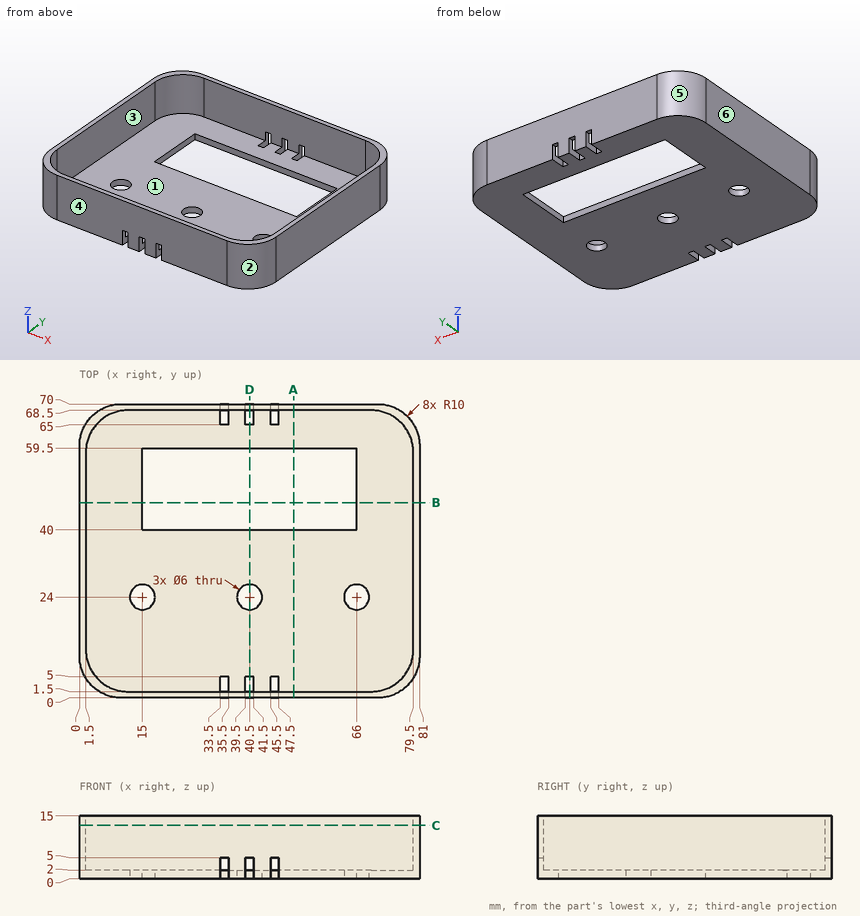
Job drawing, mm, ordinate dimensions from the low corner. One solid piece. A direction names the side the tool comes from. Coordinates: 2 decimals unless noted, no trailing zeros. Order: outer loops, then holes, each group sorted by start corner. A loop starts at its lowest first (then second) coordinate and runs counter-clockwise, first axis right, second up. Notation, with made-up numbers: (39.25, -30) -> (71.25, -30) arc R25 cw to (71.25, -9) -> close; hole circle Ø6 at (13.25, 66.5). An arc over 180 degrees is marked (long way). Return JSON: item names as keys, results as strings. Group by question number.
Item 1: Pull direction Y, two halves, no side cores. Call the marked faces 3, 4, 5 and 6: pulls with the +Y half, pulls with the -Y half, needs draft (parallel to the pull), parting line crosses it, or undercut.
Item 2: Saw through at C-C on z = 12.75. Write the cut outline in (x, y).
Item 3: Saw through at B-B on y = 46.5. Write the cut outline in (x, z).
Item 4: Wall check: line 1 along Y through (x, z) = (40.5, 0.8); line 2 along Y through (x, z) = (12, 14.25); line 3 along X through (y, z) = (11.5, 11.5). Give the ranges that are in metal, low to high. Write a range as [from, to].
Item 5: Saw through at D-D on x = 40.5. Write the cut outline in (y, z).
Item 6: Flat gauge pins, fed straight in: P1, Ø2, axis at x = 56, y = 59, coming from the -Z side; P2, Ø5.5, axis at x = 66, y = 24, coming from the -Z side; P3, Ø1.5, axis at x = 73, z = 9, coming from the -Y side; P4, Ø1.2, axis at x = 40.5, y = 69.5, coming from the -Z side. Where does each tip first touch, or does it go through?
Item 7: Saw through at A-A on x = 51. Write the cut outline in (y, z).
Item 8: Tool access for the marked faces 1 and 2: list every direction of +Z, -Z, +X, -X, +Y, -Y with a clear straight run to the whole face (end or side of a thin tool).
Values found:
{
 "1": {"face 3": "undercut", "face 4": "pulls with the -Y half", "face 5": "pulls with the +Y half", "face 6": "needs draft"},
 "2": {"outline": "(0, 10) arc R10 ccw to (10, 0) -> (71, 0) arc R10 ccw to (81, 10) -> (81, 60) arc R10 ccw to (71, 70) -> (10, 70) arc R10 ccw to (0, 60) -> close; hole (1.5, 11.5) arc R10 ccw to (11.5, 1.5) -> (69.5, 1.5) arc R10 ccw to (79.5, 11.5) -> (79.5, 58.5) arc R10 ccw to (69.5, 68.5) -> (11.5, 68.5) arc R10 ccw to (1.5, 58.5) -> close"},
 "3": {"outline": "(0, 0) -> (15, 0) -> (15, 2) -> (1.5, 2) -> (1.5, 15) -> (0, 15) -> close; (66, 0) -> (81, 0) -> (81, 15) -> (79.5, 15) -> (79.5, 2) -> (66, 2) -> close"},
 "4": {"line 1": "y = [5, 21], [27, 40], [59.5, 65]", "line 2": "y = [0, 1.5], [68.5, 70]", "line 3": "x = [0, 1.5], [79.5, 81]"},
 "5": {"outline": "(0, 5) -> (1.5, 5) -> (1.5, 15) -> (0, 15) -> close; (5, 0) -> (21, 0) -> (21, 2) -> (5, 2) -> close; (27, 0) -> (40, 0) -> (40, 2) -> (27, 2) -> close; (59.5, 0) -> (65, 0) -> (65, 2) -> (59.5, 2) -> close; (68.5, 5) -> (70, 5) -> (70, 15) -> (68.5, 15) -> close"},
 "6": {"P1": "stops at z = 0", "P2": "passes through", "P3": "stops at y = 0.08", "P4": "stops at z = 5"},
 "7": {"outline": "(0, 0) -> (40, 0) -> (40, 2) -> (1.5, 2) -> (1.5, 15) -> (0, 15) -> close; (59.5, 0) -> (70, 0) -> (70, 15) -> (68.5, 15) -> (68.5, 2) -> (59.5, 2) -> close"},
 "8": {"face 1": "+Z", "face 2": "+Z, -Z, +X, -Y"}
}
